The listing builds one solid part. Answer for the finished solid, in the listing's coordinates (mm). Coordinates: 2 decimals unless noted, no trailing zeros. Write each loop counter-clockwise with the first axis right and the second up, starting at its lowest first coordinate (ties: lowest second). Pieces come first, ordered by that corner, then holes.
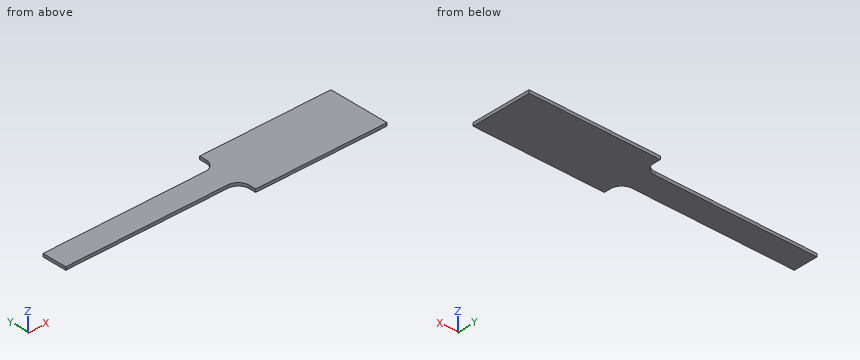
from build123d import *

# Parameters (mm, degrees)
F1_DEPTH = 1.75


with BuildPart() as f1:
    # F0 (on Top) → F1 (new body)
    with BuildSketch(Plane.XY):
        with BuildLine():
            Line((99, 3.9), (99, 0))
            Line((99, 0), (174, 0))
            Line((174, 0), (174, 34.5))
            Line((174, 34.5), (99, 34.5))
            Line((99, 34.5), (99, 30.6))
            ThreePointArc((99, 30.6), (97.1401280605, 26.1098719395), (92.65, 24.25))
            Line((92.65, 24.25), (0, 24.25))
            Line((0, 24.25), (0, 10.25))
            Line((0, 10.25), (92.65, 10.25))
            ThreePointArc((92.65, 10.25), (97.1401280605, 8.3901280605), (99, 3.9))
        make_face()
    extrude(amount=F1_DEPTH)


solid = f1.part
1. Flat-ended cylindrical pins translate along their axes: P1, Ø0.5, axis at y = 2.5, z = 0.5, coming from the -X side; P2, Ø0.5, axis at x = 30.5, z = 0.5, coming from the -Y side. Find the tip coordinate at first contact, or state that the pin passes through.
Results found:
P1: stops at x = 99
P2: stops at y = 10.25
2. Section A-A on z = 1.05 is taken. Give the vertices of the cut face in (x, y), then the cut area to 3 significant figures.
Results found:
outline: (0, 10.25) - (92.65, 10.25) arc R6.35 cw to (99, 3.9) - (99, 0) - (174, 0) - (174, 34.5) - (99, 34.5) - (99, 30.6) arc R6.35 cw to (92.65, 24.25) - (0, 24.25) - close
area: 3,990 mm2
3. Find the intervals of material crossed by L1, parallel to X at y = 30, z = 1.3; L2, parallel to Y at x = 89.5, z = 1, in increasing order.
Results found:
L1: x = 98.97 to 174
L2: y = 10.25 to 24.25
4. Section C-C on y = 8.5 is taken. Give the vertices of the cut face in (x, z).
Results found:
outline: (97.03, 0) - (174, 0) - (174, 1.75) - (97.03, 1.75) - close
5. Section B-B on x = 90.5 is taken. Give the vertices of the cut face in (y, z), then the cut area to 3 significant figures.
Results found:
outline: (10.25, 0) - (24.25, 0) - (24.25, 1.75) - (10.25, 1.75) - close
area: 24.5 mm2
